Check sheet for the modelled part. Datum: model origin and axes. Units: mm. A direction names the side the tool comes from. Coordinates: 2 decimals unless noted, no trailing zeros. Loops run counter-clockwise (first coordinate to the right, second up) from the corner with the lowest first, then second, coordinate; pieces in that order, holes last. Notation, with made-up numbers: M -21.5,26 L -8.5,26 A20 cw -8.5,63 Z; hole C 38.25,-5 d2. An arc over 180 degrees is marked long. Answer as CSV lines item,"result". Start each with the question number.
from build123d import *

# Parameters (mm, degrees)
F0_R     = 9.5
F1_DEPTH = 2.5


with BuildPart() as f1:
    # F0 (on Top) → F1 (new body)
    with BuildSketch(Plane.XY):
        with BuildLine():
            ThreePointArc((-14.330367, 68.789729), (-2.241038, 49.526311), (15, 64.357958))
            ThreePointArc((15, 64.357958), (14.831647, 66.598995), (14.330367, 68.789729))
            ThreePointArc((14.330367, 68.789729), (0, 79.357958), (-14.330367, 68.789729))
        make_face()
        with Locations((0, 64.357958)):
            Circle(F0_R, mode=Mode.SUBTRACT)
        with BuildLine():
            ThreePointArc((14.330367, 68.789729), (14.831647, 66.598995), (15, 64.357958))
            ThreePointArc((15, 64.357958), (-2.241038, 49.526311), (-14.330367, 68.789729))
            Line((-14.330367, 68.789729), (-55.684302, -64.930417))
            Line((-55.684302, -64.930417), (-55.684302, -77.022406))
            ThreePointArc((-55.684302, -77.022406), (-54.805622, -79.143726), (-52.684302, -80.022406))
            Line((-52.684302, -80.022406), (-36.684302, -80.022406))
            ThreePointArc((-36.684302, -80.022406), (-34.562982, -79.143726), (-33.684302, -77.022406))
            Line((-33.684302, -77.022406), (-33.684302, -64.930417))
            Line((-33.684302, -64.930417), (33.684302, -64.930417))
            Line((33.684302, -64.930417), (33.684302, -77.022406))
            ThreePointArc((33.684302, -77.022406), (34.562982, -79.143726), (36.684302, -80.022406))
            Line((36.684302, -80.022406), (52.684302, -80.022406))
            ThreePointArc((52.684302, -80.022406), (54.805622, -79.143726), (55.684302, -77.022406))
            Line((55.684302, -77.022406), (55.684302, -64.930417))
            Line((55.684302, -64.930417), (14.330367, 68.789729))
        make_face()
        Polygon((33.684302, -49.930417), (0, -49.930417), (-33.684302, -49.930417), (0, 46.357958), align=None, mode=Mode.SUBTRACT)
    extrude(amount=F1_DEPTH)


solid = f1.part
Item 1: Sectioned sample at A-A, the plane z = 1.3. Record the boundary of the cut face in (x, y), and give its area (3 significant figures).
Item 2: Set-up check for faces 4 (the face through (-54.83, -79.12, 1.23)), 5 (the face through (-34.59, -79.17, 1.23)), 6 (the face through (-17.078, -2.46, 1.232)): record each of +Z, -Z, +X, -X, +Y, -Y from which the full face is reachable in a straight line by a thin tool's end or side.
Item 3: Release check for a two-part mould opening along Y. For faces 1 (the face through (16.6, -1.1, 1.2)), 2 (the face through (0.267, 79.356, 1.232)), 3 (the face through (34.54, -79.12, 1.23)) record: released by +Y, released by -Y, zero draft, split by the parting line, or undercut.
Item 4: Sectioned sample at C-C, the plane x = 24. Record the boundary of the cut face in (y, z), and give its area (3 significant figures).
Item 5: Sectioned sample at B-B, the plane x = -23. Record the boundary of the cut face in (y, z).
Item 6: Go/stop test with flat-tipped pins: pin 1 (24.5 mm diameter, centred on x = 0, y = 64.36, fed in from +Z); pin 2 (1 mm diameter, centred on x = -31.5, z = 1, fed in from -Y). Record where each tip stops, or that it passes through.
Item 7: Material ranges on line 1 (X direction, y = 1.5, z = 1.2); line 2 (X direction, y = 46, z = 1.55); line 3 (X direction, y = 50.5, z = 1.4), recorded low to high. Write a range as from..to.
Item 8: Sectioned sample at D-D, the plane x = -46.5. Record the boundary of the cut face in (y, z).
Reply:
1,outline,"M -55.68,-77.02 A3 ccw -52.68,-80.02 L -36.68,-80.02 A3 ccw -33.68,-77.02 L -33.68,-64.93 L 33.68,-64.93 L 33.68,-77.02 A3 ccw 36.68,-80.02 L 52.68,-80.02 A3 ccw 55.68,-77.02 L 55.68,-64.93 L 14.33,68.79 A15 ccw -14.33,68.79 L -55.68,-64.93 Z; hole M -33.68,-49.93 L 33.68,-49.93 L 0,46.36 Z; hole C 0,64.36 d19"
1,area,"6,710 mm²"
2,face 4,"+Z, -Z, -X, -Y"
2,face 5,"+Z, -Z, -Y"
2,face 6,"+Z, -Z"
3,face 1,"undercut"
3,face 2,"released by +Y"
3,face 3,"released by -Y"
4,outline,"M -64.93,0 L -49.93,0 L -49.93,2.5 L -64.93,2.5 Z; M -22.25,0 L 37.52,0 L 37.52,2.5 L -22.25,2.5 Z"
4,area,"187 mm²"
5,outline,"M -64.93,0 L -49.93,0 L -49.93,2.5 L -64.93,2.5 Z; M -19.39,0 L 40.76,0 L 40.76,2.5 L -19.39,2.5 Z"
6,pin 1,"z = 2.5"
6,pin 2,"y = -64.93"
7,line 1,"-35.14..-15.69, 15.69..35.14"
7,line 2,"-21.38..-0.13, 0.13..21.38"
7,line 3,"-19.99..19.99"
8,outline,"M -80.02,0 L -35.23,0 L -35.23,2.5 L -80.02,2.5 Z"
